Could you check a few things on this model? Use its own coordinates, in mm. Face numbers are marked on the shaded views. Coordinates: 2 decimals unless noted, no trailing zeros. Loops run counter-clockwise (first coordinate to the right, second up) from the corner with the lowest first, then second, coordinate; pieces in that order, holes last. Notation, with made-up numbers: (28, 70.5) - (87, 70.5) arc R16 cw to (87, 94.5) - close; hole circle Ø1 at (12, 11.25). An arc over 180 degrees is marked (long way). One line per item, written item: value. Start each with the question number.
(1) If we section it at A-A on y = -40.5: Write out the boundary of the cut face in (x, z).
(2) If we section it at B-B on x = -151: Write out the boundary of the cut face in (y, z), then the cut area to 3 significant figures.
(3) I'm going to push flat-ended pins straight in: P1, Ø4, axis at x = -140, z = 12.5, coming from the +Y side; P2, Ø1, axis at y = -24.5, z = 17, coming from the -X side; P3, Ø8, axis at y = 79.5, z = 2.5, coming from the +X side; P4, Ø12, axis at x = -32, y = -38, coming from the -Z side. Where does each tip first touch, or does it pass through?
(4) If I drill on line 1 along X through (y, z) = (-54.5, 2.25); line 2 along X through (y, z) = (-61, 8.25); line 3 along Y through (x, z) = (130, 8.5), over which ranges is the centre line in solid material (lowest first)? Write a range as from..to.
(5) If we mould it in two halves opening along X, with no side actions, what happens to the marked faces 1, 2 and 3? For each: pulls with the +X half, pulls with the -X half, needs draft (parallel to the pull), parting line crosses it, or undercut.
```python
from build123d import *

# Parameters (mm, degrees)
F0_W     = 400
F0_H     = 350
F1_DEPTH = 19
F2_W     = 400
F2_H     = 350
F3_DEPTH = 19.001
F4_R     = 38.0303111514
F5_DEPTH = 19.0010001


with BuildPart() as f1:
    # F0 (on Top) → F1 (new body)
    with BuildSketch(Plane.XY):
        Rectangle(F0_W, F0_H)
    extrude(amount=F1_DEPTH)

    # F2 (on face) → F3 (cut, through all)
    with BuildSketch(Plane.XY.offset(19)):
        Rectangle(F2_W, F2_H)
        with BuildLine():
            ThreePointArc((158.4707796574, -100.301399827), (-82.4477385445, -142.2049434954), (-181.7189997485, 81.2740400434))
            ThreePointArc((-181.7189997485, 81.2740400434), (-85.5590162079, 156.2453408499), (10.6009673327, 81.2740400434))
            add(Edge.make_bspline(
                [(10.6009673327, 81.2740400434), (12.0537158036, 71.790848631), (15.059544227, 52.1997014281), (37.4294986076, 35.9210738365), (59.8496179692, 20.1880319647), (91.7535141562, 16.7841239745), (121.2377669037, 21.3632017782), (139.2062429445, 19.1287691589), (155.2089601755, 13.8627961278), (166.6253805161, 0)],
                knots=[0, 0, 0, 0, 0.1451383216, 0.28483723, 0.426890771, 0.5810119484, 0.7292272805, 0.8398242455, 1, 1, 1, 1], degree=3))
            ThreePointArc((166.6253805161, 0), (185.9978425352, -52.0571882908), (158.4707796574, -100.301399827))
        make_face(mode=Mode.SUBTRACT)
    extrude(amount=-F3_DEPTH, mode=Mode.SUBTRACT)

    # F4 (on face) → F5 (cut, through all)
    with BuildSketch(Plane.XY.offset(19)):
        with Locations((120.645708, -46.7439965176)):
            Circle(F4_R)
    extrude(amount=-F5_DEPTH, mode=Mode.SUBTRACT)


solid = f1.part
```
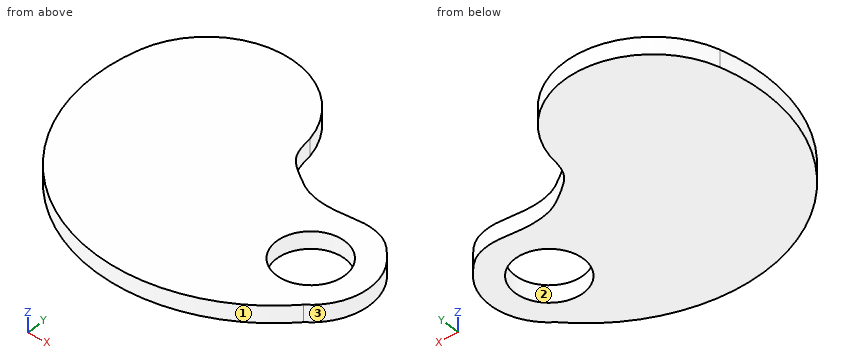
Values:
1. outline: (-173.48, 0) - (83.13, 0) - (83.13, 19) - (-173.48, 19) - close; (158.16, 0) - (185.92, 0) - (185.92, 19) - (158.16, 19) - close
2. outline: (-81.82, 0) - (131.58, 0) - (131.58, 19) - (-81.82, 19) - close
2. area: 4,050 mm2
3. P1: stops at y = 141.24
3. P2: stops at x = -179.23
3. P3: stops at x = 11.51
3. P4: stops at z = 0
4. line 1: x = -167.26..83.41, 157.88..185.75
4. line 2: x = -163.91..85.39, 155.9..184.64
4. line 3: y = -126.18..-83.61, -9.88..20.09
5. face 1: parting line crosses it
5. face 2: undercut
5. face 3: pulls with the +X half
